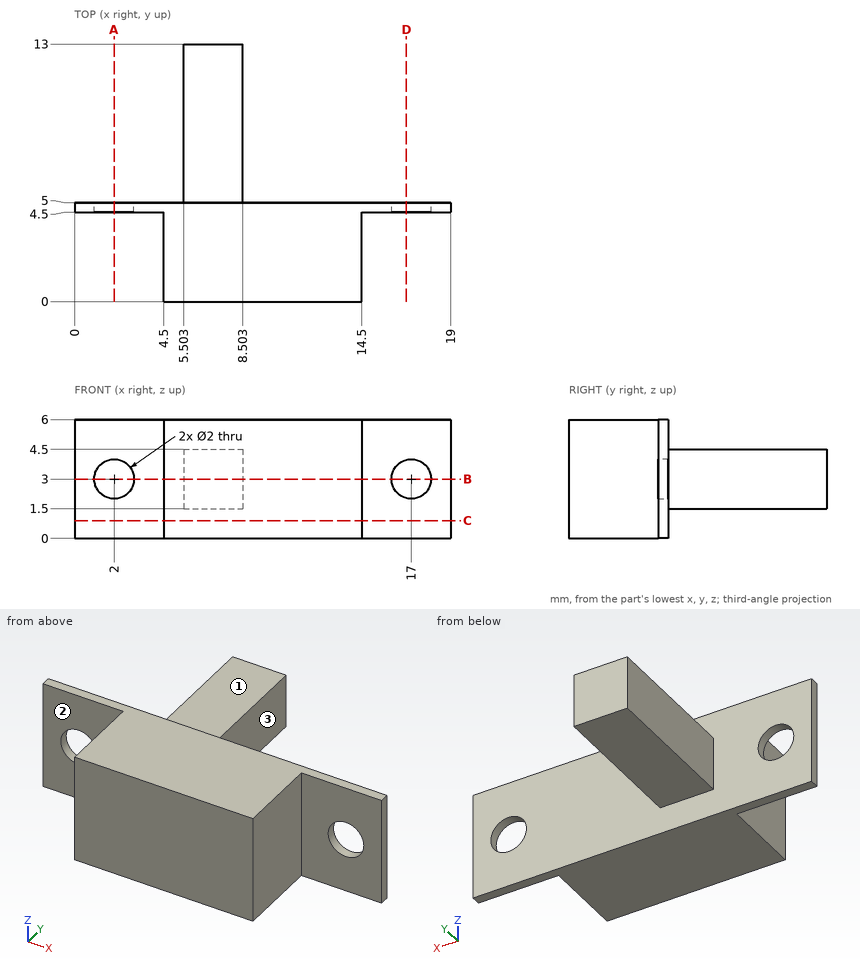
Job drawing, mm, ordinate dimensions from the low corner. One solid piece. A direction names the side the tool comes from. Round coordinates to 2 decimals unless told otherwise and drop trailing zeros. Write each loop counter-clockwise with the first axis right and the second up, starting at its lowest first coordinate (ties: lowest second). Pieces come first, ordered by that corner, then holes. Notation, with made-up numbers: M 79.5,-2.5 L 114.5,-2.5 A29 cw 114.5,28.5 Z; hole C -38.75,75 d2. An arc over 180 degrees is marked long. Return JSON: item names as keys, results as strings. Group by question number.
(1) Drill centre lines: probe 1 along X at (y, z) = (4.6, 3); probe 2 along Y at (x, z) = (12, 3.95); probe 3 along X at (y, z) = (0.75, 4.2). Where is each one in solid material? Low to high.
(2) Saw through at B-B on z = 3. Write the cut outline in (x, y).
(3) Pin check, flat tips, straight feed: pin 1 Ø1.5 at (x, z) = (12, 1.5) entering from -Y; pin 2 Ø1.5 at (x, y) = (7, 10) entering from -Z; pin 3 Ø2.5 at (x, z) = (2, 3) entering from -Y; pin 4 Ø0.9 at (y, z) = (9, 2.5) entering from +X. Stop position of each tip, or through.
(4) Saw through at A-A on x = 2. Write the cut outline in (y, z), then the cut area to 3 significant figures.
(5) Saw through at D-D on x = 16.75. Write the cut outline in (y, z).
(6) Saw through at C-C on z = 0.9. Write the cut outline in (x, y), then the cut area to 3 significant figures.
(7) Which spindle directions (+Z, -Z, +X, -X, +Y, -Y) get a long thin tool onto all of the face, cutting with end or side? Do the marked faces 1, 2 and 3. Say none if no direction does.
Returned:
{
 "1": {"probe 1": "0 to 1, 3 to 16, 18 to 19", "probe 2": "0 to 5", "probe 3": "4.5 to 14.5"},
 "2": {"outline": "M 0,4.5 L 1,4.5 L 1,5 L 0,5 Z; M 3,4.5 L 4.5,4.5 L 4.5,0 L 14.5,0 L 14.5,4.5 L 16,4.5 L 16,5 L 8.5,5 L 8.5,13 L 5.5,13 L 5.5,5 L 3,5 Z; M 18,4.5 L 19,4.5 L 19,5 L 18,5 Z"},
 "3": {"pin 1": "y = 0", "pin 2": "z = 1.5", "pin 3": "y = 4.5", "pin 4": "x = 8.5"},
 "4": {"outline": "M 4.5,0 L 5,0 L 5,2 L 4.5,2 Z; M 4.5,4 L 5,4 L 5,6 L 4.5,6 Z", "area": "2.00 mm²"},
 "5": {"outline": "M 4.5,0 L 5,0 L 5,2.03 L 4.5,2.03 Z; M 4.5,3.97 L 5,3.97 L 5,6 L 4.5,6 Z"},
 "6": {"outline": "M 0,4.5 L 4.5,4.5 L 4.5,0 L 14.5,0 L 14.5,4.5 L 19,4.5 L 19,5 L 0,5 Z", "area": "54.5 mm²"},
 "7": {"face 1": "+Z, +X, -X, +Y", "face 2": "+Z, -Z, -X, -Y", "face 3": "+Z, -Z, +X, +Y"}
}
